from build123d import *

# Parameters (mm, degrees)
SKETCH1_W           = 161.892
SKETCH1_H           = 175.354
BOSS_EXTRUDE1_DEPTH = 5
SKETCH2_W           = 17
SKETCH2_H           = 17
BOSS_EXTRUDE2_DEPTH = 3.5
SKETCH3_R           = 0.8
CUT_EXTRUDE1_DEPTH  = 120.63177356
FILLET1_R           = 2.5
CHAMFER1_SIZE       = 0.3


with BuildPart() as part:
    # Sketch1 → Boss-Extrude1 (new body)
    with BuildSketch(Plane(origin=(0, 0, 0), x_dir=(0, 1, 0), z_dir=(0, 0, 1))):
        Rectangle(SKETCH1_W, SKETCH1_H)
    extrude(amount=BOSS_EXTRUDE1_DEPTH)

    # Sketch2 → Boss-Extrude2 (add)
    with BuildSketch(Plane.XY.offset(5)):
        with Locations((79.177, 72.446)):
            Rectangle(SKETCH2_W, SKETCH2_H)
        with Locations((79.177, -72.446)):
            Rectangle(SKETCH2_W, SKETCH2_H)
        with Locations((-79.177, -72.446)):
            Rectangle(SKETCH2_W, SKETCH2_H)
        with Locations((-79.177, 72.446)):
            Rectangle(SKETCH2_W, SKETCH2_H)
    extrude(amount=BOSS_EXTRUDE2_DEPTH)

    # Sketch3 → Cut-Extrude1 (cut, through all)
    with BuildSketch(Plane.XY.offset(8.5)):
        with Locations((-76.2, 69.596)):
            Circle(SKETCH3_R)
        with Locations((76.2, 69.596)):
            Circle(SKETCH3_R)
        with Locations((76.2, -69.596)):
            Circle(SKETCH3_R)
        with Locations((-76.2, -69.596)):
            Circle(SKETCH3_R)
    extrude(amount=-CUT_EXTRUDE1_DEPTH, mode=Mode.SUBTRACT)

    # Fillet1
    fillet1_edges = [part.edges().sort_by_distance(p)[0] for p in [
        (-70.677, 63.946, 6.75),
        (70.677, 63.946, 6.75),
        (70.677, -63.946, 6.75),
        (-70.677, -63.946, 6.75),
    ]]
    fillet(fillet1_edges, radius=FILLET1_R)

    # Chamfer1
    chamfer1_edges = [part.edges().sort_by_distance(p)[0] for p in [
        (87.677, 0, 0),
        (0, -80.946, 0),
        (-87.677, 0, 0),
        (0, 80.946, 0),
        (-77, -69.596, 0),
        (75.4, -69.596, 0),
        (75.4, 69.596, 0),
        (-77, 69.596, 0),
    ]]
    chamfer(chamfer1_edges, length=CHAMFER1_SIZE)


solid = part.part
Geometry: final body of the model. Coordinates: model frame, mm. Give positions to 0.01 mm unless a question says otherwise; leave off trailing zeros. Write each loop counter-clockwise with the first axis right and the second up, starting at its lowest first coordinate (ties: lowest second). Pieces come first, ordered by that corner, then holes. Notation, with made-up numbers: M 74.25,14.25 L 113.25,14.25 A19 cw 113.25,29.25 Z; hole C 87.25,78.25 d10. An arc over 180 degrees is marked long. Answer in a Markdown table with one row per item. Add a question column.
(1) Section C-C on x = 24. Return loops of the section in (y, z).
(2) Section A-A on z = 7. Return loops of the section in (x, y).
(3) Ray query, line 1 (Y direction, x = 76.2, z = 3.5); line 2 (X direction, y = -71.5, z = 5.75); line 3 (Y direction, x = -74, z = 5.25). Return the intervals inside material, ascending.
(4) Mould query, pull axis Y, two halves, no side actions, for faces 1 (the flat face through (-1, 80.946, 3)), 2 (the flat face through (-87.677, -1, 3)), 3 (the flat face through (-1, -1, 5)). Classes: +Y half, -Y half, draft (parallel to the pull), parting line (faces both ways), or undercut.
(5) Section B-B on y = -9. Return loops of the section in (x, z).
Result set:
| question | item | result |
|---|---|---|
| 1 | outline | M -80.95,0.3 L -80.65,0 L 80.65,0 L 80.95,0.3 L 80.95,5 L -80.95,5 Z |
| 2 | outline | M -87.68,-80.95 L -70.68,-80.95 L -70.68,-66.45 A2.5 ccw -73.18,-63.95 L -87.68,-63.95 Z; M -87.68,63.95 L -73.18,63.95 A2.5 ccw -70.68,66.45 L -70.68,80.95 L -87.68,80.95 Z; M 70.68,-80.95 L 87.68,-80.95 L 87.68,-63.95 L 73.18,-63.95 A2.5 ccw 70.68,-66.45 Z; M 70.68,66.45 A2.5 ccw 73.18,63.95 L 87.68,63.95 L 87.68,80.95 L 70.68,80.95 Z; hole C -76.2,-69.6 d1.6; hole C -76.2,69.6 d1.6; hole C 76.2,-69.6 d1.6; hole C 76.2,69.6 d1.6 |
| 3 | line 1 | y = -80.95 to -70.4, -68.8 to 68.8, 70.4 to 80.95 |
| 3 | line 2 | x = -87.68 to -70.68, 70.68 to 87.68 |
| 3 | line 3 | y = -80.95 to -63.95, 63.95 to 80.95 |
| 4 | face 1 | +Y half |
| 4 | face 2 | draft |
| 4 | face 3 | undercut |
| 5 | outline | M -87.68,0.3 L -87.38,0 L 87.38,0 L 87.68,0.3 L 87.68,5 L -87.68,5 Z |
